Could you check a few things on this model? Use its own coordinates, in mm. Face numbers are marked on the shaded views. A direction names the side the tool comes from. Give positions to 0.01 mm unless a question says otherwise; leave off trailing zeros. Order: outer loops, then holes, each group sorted by start corner. A loop starts at its lowest first (then second) coordinate and runs counter-clockwise, first axis right, second up. Notation, with made-up numbers: M 33,-29.75 L 51,-29.75 A22 ccw 51,-13.75 Z; hole C 38,-7 d4. An arc over 180 degrees is marked long. Use a Markdown table: item, result. Add a question column.
Item 1: Suppose I cut it at D-D on y = -30.5. Write out the boundary of the cut face in (x, z).
Item 2: Suppose I cut it at A-A on x = -19. Write out the boundary of the cut face in (y, z).
Item 3: For the marked faces 1, 2 and 3, which set-ups out of +Z, -Z, +X, -X, +Y, -Y let a thin tool reach every point of the face, with its end or its side?
Item 4: If I drill on L1, parallel to X at y = -66.5, z = 147; L2, parallel to X at y = -66.5, z = -36; L3, parallel to Z at x = -171, y = -63, over which ranges is the centre line in solid material (lowest first)? Write a range as from..to.
Item 5: Suppose I cut it at B-B on y = -112. Write out the boundary of the cut face in (x, z), plus the area to 3 significant figures.
Item 6: Suppose I cut it at C-C on x = -179. Write out the boundary of the cut face in (y, z).
Item 7: I'm going to push flat-ended pins straight in: pin 1 Ø4 at (y, z) = (-77.5, 4.5) entering from -X; pin 2 Ø1 at (x, y) = (-91, -40.5) entering from +Z; pin 3 Ø1.5 at (x, y) = (-165, -84.5) entering from +Z. Where does each tip first touch, or does it pass through?
Item 8: If we mould it in two halves opening along X, with no side actions, what happens to the marked faces 4, 5, 6 and 7? For each: released by +X, released by -X, zero draft, split by the parting line, or undercut.
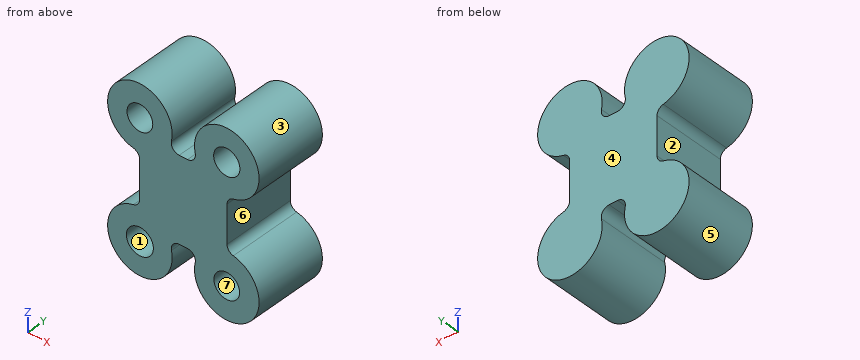
from build123d import *

# Parameters (mm, degrees)
F1_DEPTH = 118.872
F2_R     = 12.7
F5_R     = 20.788829
F5_R_2   = 21.17652
F5_R_3   = 20.68959
F5_R_4   = 21.770913
F6_DEPTH = 71.628


with BuildPart() as f1:
    # F0 (on Front) → F1 (new body)
    with BuildSketch(Plane.XZ):
        with BuildLine():
            Line((-48.653666, 52.151624), (-119.223386, 52.151624))
            Line((-119.223386, 52.151624), (-119.223386, -15.579229))
            Line((-119.223386, -15.579229), (-94.042334, -15.579229))
            ThreePointArc((-94.042334, -15.579229), (-23.388954, -87.372558), (-48.653666, 10.135782))
            Line((-48.653666, 10.135782), (-48.653666, 52.151624))
        make_face()
    extrude(amount=F1_DEPTH)

    # F2
    f2_edges = [f1.edges().sort_by_distance(p)[0] for p in [
        (-94.042334, -59.436, -15.579229),
        (-48.653666, -59.436, 10.135782),
    ]]
    fillet(f2_edges, radius=F2_R)

    # F3: F1 across face


with BuildPart() as f1_1:
    add(f1.part)
    add(f1.part.mirror(Plane(origin=(-119.223386, -59.436, 18.286197), x_dir=(0, -1, 0), z_dir=(-1, 0, 0))))

    # F4: F1 across face


with BuildPart() as f1_2:
    add(f1_1.part)
    add(f1_1.part.mirror(Plane(origin=(-119.223386, -59.436, 52.151624), x_dir=(1, 0, 0), z_dir=(0, 0, 1))))

    # F5 (on face) → F6 (cut)
    with BuildSketch(Plane.XZ.offset(118.872)):
        with Locations((-189.354789, 146.308288)):
            Circle(F5_R)
        with Locations((-49.091984, 146.308288)):
            Circle(F5_R_2)
        with Locations((-49.091984, -42.00504)):
            Circle(F5_R_3)
        with Locations((-189.354789, -42.00504)):
            Circle(F5_R_4)
    extrude(amount=-F6_DEPTH, mode=Mode.SUBTRACT)


solid = f1_2.part
Findings below:
| question | item | result |
|---|---|---|
| 1 | outline | M -199.92,9.06 A52.14 ccw long -138.39,-30.97 A12.7 cw -125.98,-15.58 L -112.47,-15.58 A12.7 cw -100.05,-30.97 A52.14 ccw long -38.53,9.06 A12.7 cw -48.65,21.49 L -48.65,82.81 A12.7 cw -38.53,95.25 A52.14 ccw long -100.05,135.27 A12.7 cw -112.47,119.88 L -125.98,119.88 A12.7 cw -138.39,135.27 A52.14 ccw long -199.92,95.25 A12.7 cw -189.79,82.81 L -189.79,21.49 A12.7 cw Z |
| 2 | outline | M -118.87,-84.59 L 0,-84.59 L 0,0.58 L -118.87,0.58 Z; M -118.87,103.73 L 0,103.73 L 0,188.89 L -118.87,188.89 Z |
| 3 | face 1 | -Y |
| 3 | face 2 | -X, +Y, -Y |
| 3 | face 3 | +Y, -Y |
| 4 | L1 | x = -241.49..-210.13, -168.58..-137.22, -101.23..-70.26, -27.93..3.05 |
| 4 | L2 | x = -241.15..-210.28, -168.43..-137.56, -100.89..-68.89, -29.29..2.7 |
| 4 | L3 | z = -90.81..-53.71, -30.3..136.55, 156.07..195.11 |
| 5 | outline | M -199.92,9.06 A52.14 ccw long -138.39,-30.97 A12.7 cw -125.98,-15.58 L -112.47,-15.58 A12.7 cw -100.05,-30.97 A52.14 ccw long -38.53,9.06 A12.7 cw -48.65,21.49 L -48.65,82.81 A12.7 cw -38.53,95.25 A52.14 ccw long -100.05,135.27 A12.7 cw -112.47,119.88 L -125.98,119.88 A12.7 cw -138.39,135.27 A52.14 ccw long -199.92,95.25 A12.7 cw -189.79,82.81 L -189.79,21.49 A12.7 cw Z; hole C -189.35,-42.01 d43.54; hole C -189.35,146.31 d41.58; hole C -49.09,146.31 d42.35; hole C -49.09,-42.01 d41.38 |
| 5 | area | 44,700 mm^2 |
| 6 | outline | M -118.87,-93.11 L 0,-93.11 L 0,197.41 L -118.87,197.41 L -118.87,164.33 L -47.24,164.33 L -47.24,128.28 L -118.87,128.28 L -118.87,-22.85 L -47.24,-22.85 L -47.24,-61.16 L -118.87,-61.16 Z |
| 7 | pin 1 | stops at x = -216.52 |
| 7 | pin 2 | stops at z = 178 |
| 7 | pin 3 | stops at z = 192.8 |
| 8 | face 4 | zero draft |
| 8 | face 5 | undercut |
| 8 | face 6 | released by +X |
| 8 | face 7 | undercut |
